Could you check a few things on this drawing? It's one solid part, dimensions in mm from its lowest x, y, z. A direction names the side the tool comes from. Give positions to 0.01 mm unless a question says otherwise; leave off trailing zeros. Order: outer loops, then holes, each group sorted by start corner. A loop starts at its lowest first (then second) coordinate and runs counter-clockwise, first axis right, second up. Notation, with made-up numbers: (-11.75, 6) - (14.25, 6) arc R20 ccw to (14.25, 11) - close; hole circle Ø3 at (-3, 20.25). An arc over 180 degrees is marked (long way). Answer as CSV lines item,"result".
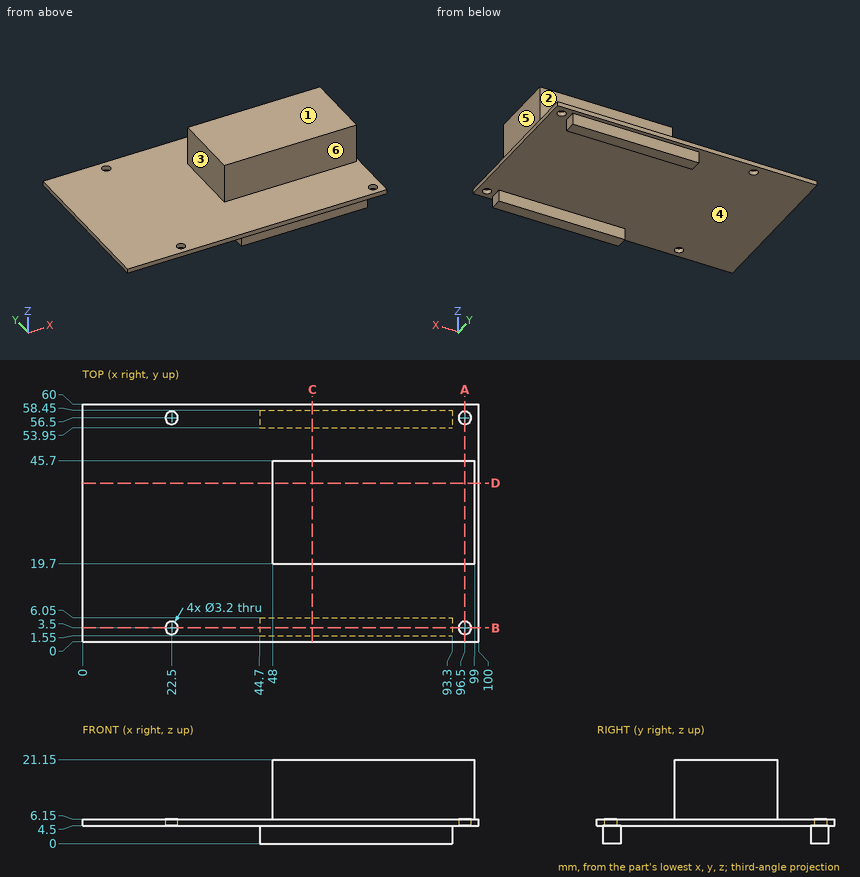
1) I want a section at C-C on x = 58. Write out the boundary of the cut face in (y, z), plus the area to 4 significant figures.
Answer block:
outline,"(0, 4.5) - (1.55, 4.5) - (1.55, 0) - (6.05, 0) - (6.05, 4.5) - (53.95, 4.5) - (53.95, 0) - (58.45, 0) - (58.45, 4.5) - (60, 4.5) - (60, 6.15) - (45.7, 6.15) - (45.7, 21.15) - (19.7, 21.15) - (19.7, 6.15) - (0, 6.15) - close"
area,"529.5 mm2"
2) I need wall thicknesses on line 1 along Y through (x, z) = (22.5, 4.9); line 2 along Y through (x, z) = (77.5, 1.5); line 3 along Y through (x, z) = (81, 18.5). Which ranges of each line are inside material? Lowest first, please. Write a range as [from, to].
Answer block:
line 1,"[0, 1.9], [5.1, 54.9], [58.1, 60]"
line 2,"[1.55, 6.05], [53.95, 58.45]"
line 3,"[19.7, 45.7]"
3) I want a section at D-D on y = 40. Write out the boundary of the cut face in (x, z), plus the area to 3 significant figures.
Answer block:
outline,"(0, 4.5) - (100, 4.5) - (100, 6.15) - (99, 6.15) - (99, 21.15) - (48, 21.15) - (48, 6.15) - (0, 6.15) - close"
area,"930 mm2"
4) If we mould it in two halves opening along Y, with no side actions, what happens to the marked faces 4, 5 and 6? For each: +Y half, -Y half, draft (parallel to the pull), parting line (faces both ways), or undercut.
Answer block:
face 4,"undercut"
face 5,"draft"
face 6,"-Y half"
5) I want a section at A-A on x = 96.5. Write out the boundary of the cut face in (y, z).
Answer block:
outline,"(0, 4.5) - (1.9, 4.5) - (1.9, 6.15) - (0, 6.15) - close; (5.1, 4.5) - (54.9, 4.5) - (54.9, 6.15) - (45.7, 6.15) - (45.7, 21.15) - (19.7, 21.15) - (19.7, 6.15) - (5.1, 6.15) - close; (58.1, 4.5) - (60, 4.5) - (60, 6.15) - (58.1, 6.15) - close"
6) I'm going to push flat-ended pins straight in: P1, Ø5, axis at y = 55.5, z = 1.5, coming from the +X side; P2, Ø1.3, axis at x = 64, z = 2.5, coming from the -Y side; P3, Ø1.9, axis at x = 96.5, y = 3.5, coming from the +Z side; P4, Ø4.5, axis at x = 62.5, z = 15, coming from the -Y side. Where does each tip first touch, or does it pass through?
Answer block:
P1,"x = 93.3"
P2,"y = 1.55"
P3,"through"
P4,"y = 19.7"
7) I want a section at B-B on y = 3.5. Write out the boundary of the cut face in (x, z).
Answer block:
outline,"(0, 4.5) - (20.9, 4.5) - (20.9, 6.15) - (0, 6.15) - close; (24.1, 4.5) - (44.7, 4.5) - (44.7, 0) - (93.3, 0) - (93.3, 4.5) - (94.9, 4.5) - (94.9, 6.15) - (24.1, 6.15) - close; (98.1, 4.5) - (100, 4.5) - (100, 6.15) - (98.1, 6.15) - close"
8) Which directions (+Z, -Z, +X, -X, +Y, -Y) give clear straight access to the entire face, cutting with the end or side of a thin tool? Please do the marked faces 1, 2 and 3.
Answer block:
face 1,"+Z, +X, -X, +Y, -Y"
face 2,"+Z, +X, -X, +Y"
face 3,"+Z, -X, +Y, -Y"
